For this review, use the dimensioned drawing (mm, ordinates from the lowest corner) and the shaded views. A direction names the side the tool comes from. Give positions to 0.01 mm unless a question says otherwise; leave off trailing zeros. Write each loop counter-clockwise with the first axis right and the second up, starting at its lowest first coordinate (ties: lowest second). Pieces come first, ordered by that corner, then holes.
1) We need section A-A on y = 28.5. Give the boundary of the cut face in (x, z), and give its area (3 significant figures).
2) For P1, Ø1.6, axis at x = 17.5, y = 2, coming from the -Z side; P2, Ø4, axis at y = 46, z = 43.5, coming from the +X side; P3, Ø2.5, axis at y = 24.5, z = 6.5, coming from the +X side; P4, Ø12, axis at y = 39, z = 18, coming from the -X side, all flat-tipped, find the tip position at first contact; note any pin that passes through.
3) Wall thickness on line 1 along Z through (x, y) = (25, 45.5) (1 decimal); line 2 along Y through (x, z) = (21, 14); line 3 along Z through (x, y) = (11.5, 28.5): over which ranges is each line inside the solid? List them lowest first.
4) Machinability: for the marked faces 1, 2, 3 and 4, which of the approach directions +Z, -Z, +X, -X, +Y, -Y give a long, thin tool a straight path to every point of the face, cutting with its end or side? Answer none if there is none.
5) We need section B-B on x = 17.5. Give the boundary of the cut face in (y, z) (1 decimal), and give its area (3 significant figures).
6) We need section D-D on x = 7. Give the boundary of the cut face in (y, z) (1 decimal), and give its area (3 significant figures).
7) We need section C-C on z = 29.5. Give the boundary of the cut face in (x, y).
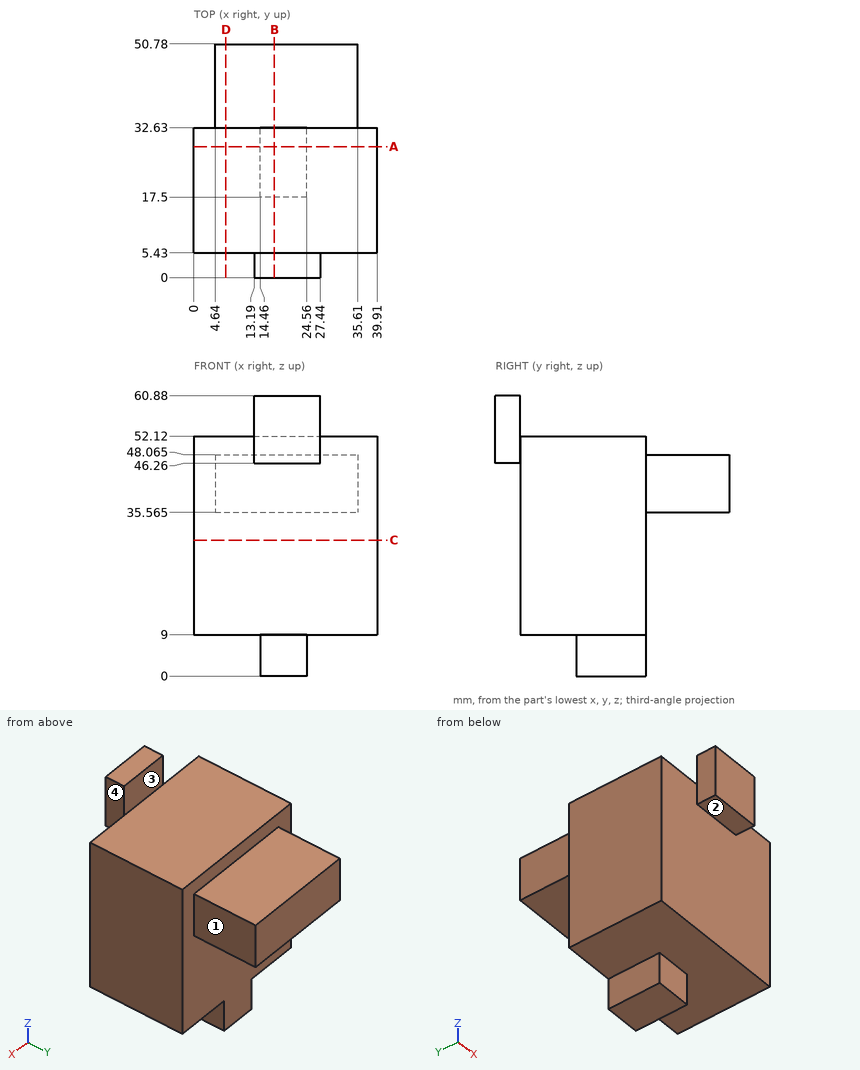
Results list:
1. outline: (0, 9) - (14.46, 9) - (14.46, 0) - (24.56, 0) - (24.56, 9) - (39.91, 9) - (39.91, 52.12) - (0, 52.12) - close
1. area: 1,810 mm2
2. P1: stops at z = 46.26
2. P2: stops at x = 35.61
2. P3: stops at x = 24.56
2. P4: passes through
3. line 1: z = 35.6 to 48.1
3. line 2: y = 5.43 to 32.63
3. line 3: z = 9 to 52.12
4. face 1: +Z, -Z, +X, +Y
4. face 2: -Z, +X, -X, -Y
4. face 3: +Z, +X, -X, +Y
4. face 4: +Z, -Z, +X, -Y
5. outline: (0, 46.3) - (5.4, 46.3) - (5.4, 9) - (17.5, 9) - (17.5, 0) - (32.6, 0) - (32.6, 35.6) - (50.8, 35.6) - (50.8, 48.1) - (32.6, 48.1) - (32.6, 52.1) - (5.4, 52.1) - (5.4, 60.9) - (0, 60.9) - close
5. area: 1,620 mm2
6. outline: (5.4, 9) - (32.6, 9) - (32.6, 35.6) - (50.8, 35.6) - (50.8, 48.1) - (32.6, 48.1) - (32.6, 52.1) - (5.4, 52.1) - close
6. area: 1,400 mm2
7. outline: (0, 5.43) - (39.91, 5.43) - (39.91, 32.63) - (0, 32.63) - close
